Geometry: final body of the model. Coordinates: model frame, mm. Face numbers are marked on the shaded views. A direction names the side the tool comes from. Round coordinates to 2 decimals unless told otherwise and drop trailing zeros. Write each loop counter-clockwise with the first axis right and the second up, starting at its lowest first coordinate (ties: lowest second). Pieces come first, ordered by that corner, then holes. Notation, with made-up numbers: (8, 42.5) - (38, 42.5) arc R25 cw to (38, 76.5) - close; hole circle Ø11 at (48, 6). An arc over 180 degrees is marked (long way). Write each question's results on one line, items separated by ' | '.
from build123d import *

# Parameters (mm, degrees)
SKETCH1_R               = 12.7
BOSS_EXTRUDE1_DEPTH     = 15.24
SKETCH2_R               = 2.9845
CUT_EXTRUDE1_DEPTH      = 7.62
SKETCH3_R               = 6.35
CUT_EXTRUDE2_DEPTH      = 7.62
CUT_EXTRUDE3_REACH      = 25.555
SKETCH7_W               = 0.635
SKETCH7_H               = 13.97
CUT_EXTRUDE4_DEPTH      = 24.727682277
CUT_EXTRUDE4_DEPTH_BACK = 24.727682277
SKETCH8_R               = 2.0955
SKETCH9_R               = 3.429
CUT_EXTRUDE5_DEPTH      = 7.62
CUT_EXTRUDE6_DEPTH      = 27.512980205


with BuildPart() as part:
    # Sketch1 → Boss-Extrude1 (new body)
    with BuildSketch(Plane.XY):
        with Locations(Location((0, 0, 0), (0, 0, 180))):
            Circle(SKETCH1_R)
    extrude(amount=BOSS_EXTRUDE1_DEPTH)

    # Sketch2 → Cut-Extrude1 (cut)
    with BuildSketch(Plane(origin=(0, 0, 0), x_dir=(-1, 0, 0), z_dir=(0, 0, -1))):
        Circle(SKETCH2_R)
    extrude(amount=-CUT_EXTRUDE1_DEPTH, mode=Mode.SUBTRACT)

    # Sketch3 → Cut-Extrude2 (cut)
    with BuildSketch(Plane.XY.offset(15.24)):
        Circle(SKETCH3_R)
    extrude(amount=-CUT_EXTRUDE2_DEPTH, mode=Mode.SUBTRACT)

    # Sketch7 → Cut-Extrude3 (cut, up to next)
    with BuildSketch(Plane(origin=(0, 0, 0), x_dir=(-1, 0, 0), z_dir=(0, 0, -1)), mode=Mode.PRIVATE) as cut_extrude3_sk1:
        with Locations((0, 6.35)):
            Rectangle(SKETCH7_W, SKETCH7_H)
    cut_extrude3_tool1 = extrude(cut_extrude3_sk1.sketch, amount=-CUT_EXTRUDE3_REACH, mode=Mode.PRIVATE) & part.part
    add(cut_extrude3_tool1.solids().sort_by_distance((0, 6.35, 0))[0], mode=Mode.SUBTRACT)

    # Sketch8 → Cut-Extrude4 (cut, two sides: drawn at the far end of the back side and taken through both)
    with BuildSketch(Plane.ZY.offset(-0.3175).offset(-CUT_EXTRUDE4_DEPTH_BACK)):
        with Locations((7.62, 9.52103063)):
            Circle(SKETCH8_R)
    extrude(amount=CUT_EXTRUDE4_DEPTH + CUT_EXTRUDE4_DEPTH_BACK, mode=Mode.SUBTRACT)

    # Sketch9 → Cut-Extrude5 (cut)
    with BuildSketch(Plane.ZY.offset(-4.8895)):
        with Locations((7.62, 9.52103063)):
            Circle(SKETCH9_R)
    extrude(amount=-CUT_EXTRUDE5_DEPTH, mode=Mode.SUBTRACT)

    # Sketch10 → Cut-Extrude6 (cut, through all)
    with BuildSketch(Plane(origin=(-4.8895, 0, 0), x_dir=(0, 0, -1), z_dir=(1, 0, 0))):
        Polygon((-10.083669069, 5.25383063), (-5.156330931, 5.25383063), (-2.692661863, 9.52103063), (-5.156330931, 13.78823063), (-10.083669069, 13.78823063), (-12.547338137, 9.52103063), align=None)
    extrude(amount=-CUT_EXTRUDE6_DEPTH, mode=Mode.SUBTRACT)


solid = part.part
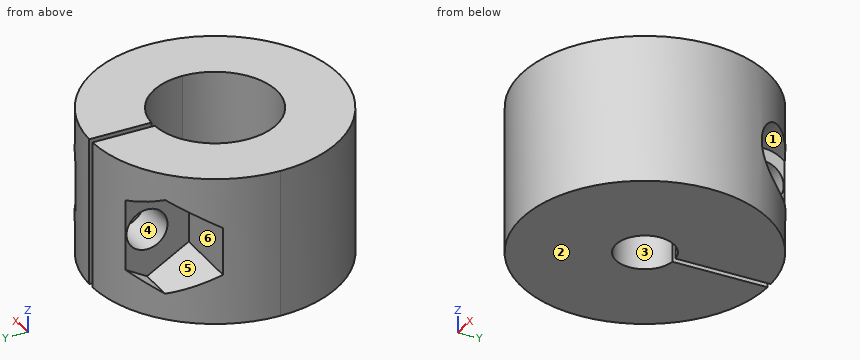
Q1. Section query A-A, the plane x = -1.25. Return loops of the section in (y, z).
Answer block:
outline: (-12.64, 0) - (-2.71, 0) - (-2.71, 7.62) - (-6.23, 7.62) - (-6.23, 15.24) - (-12.64, 15.24) - close; (2.71, 0) - (12.64, 0) - (12.64, 15.24) - (6.23, 15.24) - (6.23, 7.62) - (2.71, 7.62) - close; hole circle Ø4.19 at (9.52, 7.62)
Q2. Mould query, pull axis Z, two halves, no side actions, for the marked faces 1, 2 and 3. Classes: pulls with the +Z half, pulls with the -Z half, needs draft (parallel to the pull), parting line crosses it, or undercut.
Answer block:
face 1: undercut | face 2: pulls with the -Z half | face 3: needs draft
Q3. Pin query (flat end, axial travel): pin 1 (8 mm diameter, centred on y = 9.52, z = 7.62, fed in from +X); pin 2 (2 mm diameter, centred on y = -3.5, z = 7.5, fed in from -X); pin 3 (4 mm diameter, centred on x = -8.5, z = 7.5, fed in from -Y). Return the tip coordinate at first contact, or that it passes through.
Answer block:
pin 1: x = 11.44 | pin 2: x = -12.45 | pin 3: y = -10.91
Q4. Ray query, line 1 along X through (y, z) = (8.25, 5); line 2 along X through (y, z) = (0.25, 10.75); line 3 along Z through (x, y) = (-5.25, 1.5). Return the intervals inside material, ascending.
Answer block:
line 1: -4.89 to -0.32, 0.32 to 4.89 | line 2: -12.7 to -6.35, 6.35 to 12.7 | line 3: 0 to 7.62
Q5. Section query D-D, the plane x = -8.75. Return loops of the section in (y, z).
Answer block:
outline: (-9.2, 0) - (9.2, 0) - (9.2, 2.88) - (5.25, 5.16) - (5.25, 10.08) - (9.2, 12.36) - (9.2, 15.24) - (-9.2, 15.24) - close
Q6. Access query for the marked faces 4, 5 and 6. Directions: +Z, -Z, +X, -X, +Y, -Y. A direction counts if a zero-diameter tool reaches every point of the face in a straight line with its end or side. Return the directions, or none.
Answer block:
face 4: +X, -X | face 5: -X | face 6: -X, +Y
Q7. Section query C-C, the plane y = 10. Return loops of the section in (x, z), plus the area to 3 significant figures.
Answer block:
outline: (-7.83, 0) - (-0.32, 0) - (-0.32, 5.58) - (-4.89, 5.58) - (-4.89, 2.97) - (-7.83, 2.97) - close; (-7.83, 12.27) - (-4.89, 12.27) - (-4.89, 9.66) - (-0.32, 9.66) - (-0.32, 15.24) - (-7.83, 15.24) - close; (0.32, 0) - (7.83, 0) - (7.83, 4.22) - (4.89, 4.22) - (4.89, 5.58) - (0.32, 5.58) - close; (0.32, 9.66) - (4.89, 9.66) - (4.89, 11.02) - (7.83, 11.02) - (7.83, 15.24) - (0.32, 15.24) - close | area: 144 mm2
Q8. Section query B-B, the plane z = 8.5. Return loops of the section in (x, y), plus the area to 3 significant figures.
Answer block:
outline: (-11.56, 5.25) arc R12.7 ccw (long way) to (11.08, 6.21) - (4.89, 6.21) - (4.89, 7.62) - (0.32, 7.62) - (0.32, 6.34) arc R6.35 cw (long way) to (-0.32, 6.34) - (-0.32, 7.62) - (-4.89, 7.62) - (-4.89, 5.25) - close; (-4.89, 11.42) - (-0.32, 11.42) - (-0.32, 12.7) arc R12.7 ccw to (-4.89, 11.72) - close; (0.32, 11.42) - (4.89, 11.42) - (4.89, 11.72) arc R12.7 ccw to (0.32, 12.7) - close | area: 293 mm2
